from build123d import *

# Parameters (mm, degrees)
SKETCH1_R                    = 2.5
BASE_FLANGE1_DEPTH           = 2
EDGE_FLANGE1_STRIP_W         = 9.4732
EDGE_FLANGE1_STRIP_H         = 2
EDGE_FLANGE1_STRIP_CUT_DEPTH = 54
EDGE_FLANGE1_DEPTH           = 54
CUT_EXTRUDE1_START           = 16
CUT_EXTRUDE1_DEPTH           = 22
SKETCH10_R                   = 2.5
CUT_EXTRUDE2_DEPTH           = 10
SKETCH11_W                   = 22
SKETCH11_H                   = 17
SKETCH11_R                   = 2.5
BOSS_EXTRUDE1_DEPTH          = 2


# Read off the part's stored shape, not the designer's step: Cut-Extrude1
# Sheet-metal steps are written as plain solids
with BuildPart() as part:
    # Sketch1 → Base-Flange1 (new body)
    with BuildSketch(Plane(origin=(0, 0, 0), x_dir=(1, 0, 0), z_dir=(0, 1, 0))):
        with BuildLine():
            Line((0, 0), (54, 0))
            Line((54, 0), (54, 12.3))
            ThreePointArc((54, 12.3), (52.535533906, 15.835533906), (49, 17.3))
            Line((49, 17.3), (5, 17.3))
            ThreePointArc((5, 17.3), (1.464466094, 15.835533906), (0, 12.3))
            Line((0, 12.3), (0, 0))
        make_face()
        with Locations(Location((8, 9.3, 0), (0, 0, 270))):
            Circle(SKETCH1_R, mode=Mode.SUBTRACT)
        with Locations(Location((46, 9.3, 0), (0, 0, 90))):
            Circle(SKETCH1_R, mode=Mode.SUBTRACT)
    extrude(amount=-BASE_FLANGE1_DEPTH)

    # Edge-Flange1 strip (across the edge) → Edge-Flange1 strip cut (cut)
    with BuildSketch(Plane(origin=(0, 0, 0), x_dir=(0, 0, -1), z_dir=(1, 0, 0))):
        with Locations((-4, -1)):
            Rectangle(EDGE_FLANGE1_STRIP_W, EDGE_FLANGE1_STRIP_H)
    extrude(amount=EDGE_FLANGE1_STRIP_CUT_DEPTH, mode=Mode.SUBTRACT)

    # Edge-Flange1 section (across the edge) → Edge-Flange1 (add)
    with BuildSketch(Plane(origin=(0, 0, 0), x_dir=(0, 0, -1), z_dir=(1, 0, 0))):
        with BuildLine():
            Line((-2, 0.7366), (-2, 25))
            Line((-2, 25), (0, 25))
            Line((0, 25), (0, 0.7366))
            ThreePointArc((0, 0.7366), (0.215745145, 0.215745145), (0.7366, 0))
            Line((0.7366, 0), (0.7366, -2))
            ThreePointArc((0.7366, -2), (-1.198468417, -1.198468417), (-2, 0.7366))
        make_face()
    extrude(amount=EDGE_FLANGE1_DEPTH)

    # Cut-Extrude1 outline → Cut-Extrude1 (cut)
    with BuildSketch(Plane.YZ.offset(CUT_EXTRUDE1_START)):
        with BuildLine():
            Line((-1.899002398, 0), (0.027185133, -0.538332237))
            ThreePointArc((0.027185133, -0.538332237), (0.291327316, -0.149819123), (0.7366, 0))
            Line((0.7366, 0), (25, 0))
            Line((25, 0), (25, 2))
            Line((25, 2), (0.7366, 2))
            ThreePointArc((0.7366, 2), (-0.917667209, 1.443395312), (-1.899002398, 0))
        make_face()
    extrude(amount=CUT_EXTRUDE1_DEPTH, mode=Mode.SUBTRACT)

    # Sketch10 → Cut-Extrude2 (cut)
    with BuildSketch(Plane.XY.offset(2)):
        with BuildLine():
            ThreePointArc((46, 25), (51.656854249, 22.656854249), (54, 17))
            Line((54, 17), (54, 25))
            Line((54, 25), (46, 25))
        make_face()
        with Locations((46, 17)):
            Circle(SKETCH10_R)
        with Locations((8, 17)):
            Circle(SKETCH10_R)
        with BuildLine():
            ThreePointArc((0, 17), (2.343145728, 22.656854227), (7.999999938, 25))
            Line((7.999999938, 25), (0, 25))
            Line((0, 25), (0, 17))
        make_face()
    extrude(amount=-CUT_EXTRUDE2_DEPTH, mode=Mode.SUBTRACT)

    # Sketch11 → Boss-Extrude1 (add)
    with BuildSketch(Plane.XY.offset(2)):
        with Locations((27, 16.5)):
            Rectangle(SKETCH11_W, SKETCH11_H)
        with Locations((27, 17)):
            Circle(SKETCH11_R, mode=Mode.SUBTRACT)
    extrude(amount=-BOSS_EXTRUDE1_DEPTH)


solid = part.part
Work out the finished part from the listing and answer in its coordinate system (mm). A direction names the side the tool comes from. Round coordinates to 2 decimals unless told otherwise and drop trailing zeros. Write each loop counter-clockwise with the first axis right and the second up, starting at its lowest first coordinate (ties: lowest second). Pieces come first, ordered by that corner, then holes. Notation, with made-up numbers: (79.25, 20.25) - (136.25, 20.25) arc R17 ccw to (136.25, 32.25) - close; hole circle Ø8 at (86.5, 72). An arc over 180 degrees is marked (long way). Answer in a Markdown table with one row per item. Add a question column.
1. A cutting plane is placed at C-C, the plane z = -9.3. Determine the outline of the cut face in (x, y).
2. Given pin 1 (10 mm diameter, centred on y = 6.5, z = -12, fed in from -X); pin 2 (6 mm diameter, centred on x = 34, y = 16, fed in from -Z); pin 3 (1.6 mm diameter, centred on x = 32, z = 0.5, fed in from -Y); pin 4 (6 mm diameter, centred on x = 8, z = -9.3, fed in from +Y), each flat-ended and moving along its own axis, determine where each tip first touches the part or whether it passes through.
3. The mould has two halves that part along Z. Classify faces 4 (the cylindrical face through (5.56, -0.99, -9.84)), 5 (the flat face through (27, -1, -17.3)), 6 (the flat face through (27, -2, -9)): +Z half, -Z half, draft (parallel to the pull), parting line (faces both ways), or undercut.
4. Find the intervals of material crossed by line 1 along X through (y, z) = (-0.5, -9.3); line 2 along X through (y, z) = (2, 0.75); line 3 along X through (y, z) = (15, 0.5), in increasing order. Write a range as from..to.
5. A cutting plane is placed at A-A, the plane x = 27. Determine the outline of the cut face in (y, z), and give its area (3 significant figures).
6. For faces 1 (the flat face through (27, 8, 1)), 2 (the cylindrical face through (9.34, 19.11, 1.01)), 3 (the flat face through (27, 13, 0)), determine the directions among +Z, -Z, +X, -X, +Y, -Y from which every point of the face is accessible in a straight line to the end or side of a thin tool.
7. A cutting plane is placed at D-D, the plane x = 14.5. Determine the outline of the cut face in (y, z).
8. A cutting plane is placed at B-B, the plane y = 7. Determine the outline of the cut face in (x, z).
Worked out:
| question | item | result |
|---|---|---|
| 1 | outline | (0, -2) - (5.5, -2) - (5.5, 0) - (0, 0) - close; (10.5, -2) - (43.5, -2) - (43.5, 0) - (10.5, 0) - close; (48.5, -2) - (54, -2) - (54, 0) - (48.5, 0) - close |
| 2 | pin 1 | through |
| 2 | pin 2 | z = 0 |
| 2 | pin 3 | y = -1.96 |
| 2 | pin 4 | y = 0 |
| 3 | face 4 | undercut |
| 3 | face 5 | -Z half |
| 3 | face 6 | draft |
| 4 | line 1 | 0..5.5, 10.5..43.5, 48.5..54 |
| 4 | line 2 | 0..16, 38..54 |
| 4 | line 3 | 0..6.5, 9.5..25.5, 28.5..44.5, 47.5..54 |
| 5 | outline | (-2, -17.3) - (0, -17.3) - (0, -0.74) arc R0.74 cw to (0.03, -0.54) - (-1.9, 0) arc R2.74 ccw to (-2, -0.74) - close; (8, 0) - (14.5, 0) - (14.5, 2) - (8, 2) - close; (19.5, 0) - (25, 0) - (25, 2) - (19.5, 2) - close |
| 5 | area | 58.1 mm^2 |
| 6 | face 1 | +Z, -Z, -Y |
| 6 | face 2 | +Z, -Z |
| 6 | face 3 | -Z, +X, -X, +Y |
| 7 | outline | (-2, -17.3) - (0, -17.3) - (0, -0.74) arc R0.74 cw to (0.74, 0) - (25, 0) - (25, 2) - (0.74, 2) arc R2.74 ccw to (-2, -0.74) - close |
| 8 | outline | (0, 0) - (16, 0) - (16, 2) - (0, 2) - close; (38, 0) - (54, 0) - (54, 2) - (38, 2) - close |
